Check sheet for the modelled part. Datum: model origin and axes. Units: mm. Round coordinates to 2 decimals unless told otherwise and drop trailing zeros. Order: outer loops, then holes, each group sorted by start corner. A loop starts at its lowest first (then second) coordinate and runs counter-clockwise, first axis right, second up.
(1) Sectioned sample at C-C, the plane y = 235. Enter the section's corners in (x, z), and give its area (3 significant figures).
(2) Depth check by flat-ended pin: pin 1 (7 mm diameter, centred on x = 253.47, y = 191.47, fed in from -Z); pin 2 (3.5 mm diameter, centred on x = 20.53, y = 191.47, fed in from -Z); pin 3 (1.5 mm diameter, centred on x = 37.5, z = 1.5, fed in from +Y); pin 4 (0.9 mm diameter, centred on y = 90, z = 2, fed in from -X). Enter the tip coordinate at first touch or a pass-through.
(3) Sectioned sample at A-A, the plane x = 128. Enter the section's corners in (y, z).
(4) Sectioned sample at D-D, the plane y = 76.5. Enter the section's corners in (x, z) (3 decimals), and give its area (3 significant figures).
(5) Thickness scan on probe 1 along Y at (x, z) = (159, 1.15); probe 2 along X at (y, z) = (236.5, 0.25); probe 3 along Y at (x, z) = (57.5, 2.4). Record the ranges inside material, lowest first.
(6) Sectioned sample at B-B, the plane y = 160. Enter the section's corners in (x, z), and give its area (3 significant figures).
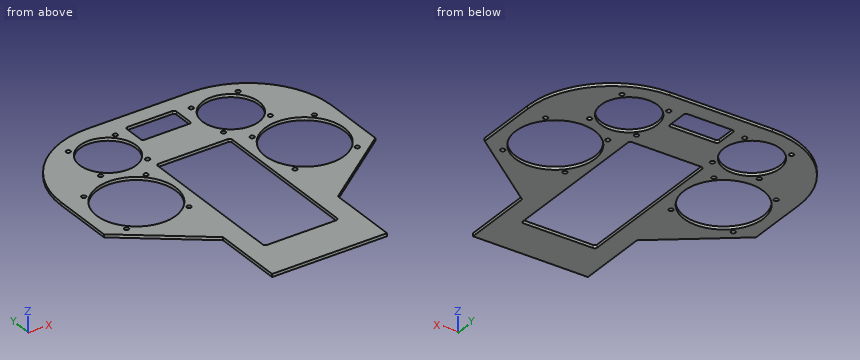
```python
from build123d import *

# Parameters (mm, degrees)
PAD_DEPTH         = 3
SKETCH001_R       = 28.5
SKETCH001_R_2     = 2.25
POCKET_DEPTH      = 3
SKETCH_R          = 40
SKETCH_R_2        = 2.25
POCKET001_DEPTH   = 3
COPYSKETCH003_R   = 40
COPYSKETCH003_R_2 = 2.25
POCKET002_DEPTH   = 5
SKETCH003_R       = 28.5
SKETCH003_R_2     = 2.25
POCKET004_DEPTH   = 5
POCKET005_DEPTH   = 5
POCKET006_DEPTH   = 5


with BuildPart() as part:
    # Sketch002 → Pad (new body)
    with BuildSketch(Plane.XY):
        with BuildLine():
            Line((0, 132), (0, 195))
            ThreePointArc((85, 280), (24.895924, 255.104076), (0, 195))
            Line((85, 280), (189, 280))
            ThreePointArc((274, 195), (249.104076, 255.104076), (189, 280))
            Line((274, 195), (274, 132))
            Line((274, 132), (195, 72))
            Line((195, 72), (195, 0))
            Line((195, 0), (79, 0))
            Line((79, 0), (79, 72))
            Line((79, 72), (0, 132))
        make_face()
    extrude(amount=PAD_DEPTH)

    # Sketch001 → Pocket (cut)
    with BuildSketch(Plane.XY):
        with Locations((75, 235)):
            Circle(SKETCH001_R)
        with Locations((98.688077, 258.688077)):
            Circle(SKETCH001_R_2)
        with Locations((51.311923, 258.688077)):
            Circle(SKETCH001_R_2)
        with Locations((51.311923, 211.311923)):
            Circle(SKETCH001_R_2)
        with Locations((98.688077, 211.311923)):
            Circle(SKETCH001_R_2)
    extrude(amount=POCKET_DEPTH, mode=Mode.SUBTRACT)

    # Sketch → Pocket001 (cut)
    with BuildSketch(Plane.XY):
        with Locations((222, 160)):
            Circle(SKETCH_R)
        with Locations((253.466252, 191.466252)):
            Circle(SKETCH_R_2)
        with Locations((190.533748, 191.466252)):
            Circle(SKETCH_R_2)
        with Locations((190.533748, 128.533748)):
            Circle(SKETCH_R_2)
        with Locations((253.466252, 128.533748)):
            Circle(SKETCH_R_2)
    extrude(amount=POCKET001_DEPTH, mode=Mode.SUBTRACT)

    # CopySketch003 → Pocket002 (cut)
    with BuildSketch(Plane.XY):
        with Locations((52, 160)):
            Circle(COPYSKETCH003_R)
        with Locations((83.466252, 191.466252)):
            Circle(COPYSKETCH003_R_2)
        with Locations((20.533748, 191.466252)):
            Circle(COPYSKETCH003_R_2)
        with Locations((20.533748, 128.533748)):
            Circle(COPYSKETCH003_R_2)
        with Locations((83.466252, 128.533748)):
            Circle(COPYSKETCH003_R_2)
    extrude(amount=POCKET002_DEPTH, mode=Mode.SUBTRACT)

    # Sketch003 → Pocket004 (cut)
    with BuildSketch(Plane.XY):
        with Locations((199, 235)):
            Circle(SKETCH003_R)
        with Locations((222.688077, 258.688077)):
            Circle(SKETCH003_R_2)
        with Locations((175.311923, 258.688077)):
            Circle(SKETCH003_R_2)
        with Locations((175.311923, 211.311923)):
            Circle(SKETCH003_R_2)
        with Locations((222.688077, 211.311923)):
            Circle(SKETCH003_R_2)
    extrude(amount=POCKET004_DEPTH, mode=Mode.SUBTRACT)

    # Sketch004 → Pocket005 (cut)
    with BuildSketch(Plane.XY):
        with BuildLine():
            Line((114.5, 263.5), (159.5, 263.5))
            ThreePointArc((162, 261), (161.267767, 262.767767), (159.5, 263.5))
            Line((162, 261), (162, 241))
            ThreePointArc((159.5, 238.5), (161.267767, 239.232233), (162, 241))
            Line((159.5, 238.5), (114.5, 238.5))
            ThreePointArc((112, 241), (112.732233, 239.232233), (114.5, 238.5))
            Line((112, 241), (112, 261))
            ThreePointArc((114.5, 263.5), (112.732233, 262.767767), (112, 261))
        make_face()
    extrude(amount=POCKET005_DEPTH, mode=Mode.SUBTRACT)

    # CopySketch005 → Pocket006 (cut)
    with BuildSketch(Plane.XY):
        with BuildLine():
            Line((102, 200), (172, 200))
            ThreePointArc((174.5, 197.5), (173.767767, 199.267767), (172, 200))
            Line((174.5, 197.5), (174.5, 43.5))
            ThreePointArc((172, 41), (173.767767, 41.732233), (174.5, 43.5))
            Line((172, 41), (102, 41))
            ThreePointArc((99.5, 43.5), (100.232233, 41.732233), (102, 41))
            Line((99.5, 43.5), (99.5, 197.5))
            ThreePointArc((102, 200), (100.232233, 199.267767), (99.5, 197.5))
        make_face()
    extrude(amount=POCKET006_DEPTH, mode=Mode.SUBTRACT)


solid = part.part
```
Derived:
1. outline: (10, 0) - (46.5, 0) - (46.5, 3) - (10, 3) - close; (103.5, 0) - (170.5, 0) - (170.5, 3) - (103.5, 3) - close; (227.5, 0) - (264, 0) - (264, 3) - (227.5, 3) - close
1. area: 420 mm2
2. pin 1: stops at z = 0
2. pin 2: passes through
2. pin 3: stops at y = 265.99
2. pin 4: stops at x = 54.71
3. outline: (0, 0) - (41, 0) - (41, 3) - (0, 3) - close; (200, 0) - (238.5, 0) - (238.5, 3) - (200, 3) - close; (263.5, 0) - (280, 0) - (280, 3) - (263.5, 3) - close
4. outline: (73.075, 0) - (99.5, 0) - (99.5, 3) - (73.075, 3) - close; (174.5, 0) - (200.925, 0) - (200.925, 3) - (174.5, 3) - close
4. area: 159 mm2
5. probe 1: y = 0 to 41, 200 to 238.5, 263.5 to 280
5. probe 2: x = 10.82 to 46.54, 103.46 to 170.54, 227.46 to 263.18
5. probe 3: y = 88.33 to 120.38, 199.62 to 212.51, 257.49 to 275.43
6. outline: (0, 0) - (12, 0) - (12, 3) - (0, 3) - close; (92, 0) - (99.5, 0) - (99.5, 3) - (92, 3) - close; (174.5, 0) - (182, 0) - (182, 3) - (174.5, 3) - close; (262, 0) - (274, 0) - (274, 3) - (262, 3) - close
6. area: 117 mm2
